Check sheet for the drawn part. Datum: minimum x, y, z corner. Units: mm. A direction names the side the tool comes from. Give positions to 0.01 mm unless a question says otherwise; leave off trailing zeros. Order: outer loops, then holes, each group sorted by start corner. A loop starts at its lowest first (then second) coordinate and runs counter-clockwise, first axis right, second up. Notation, with made-up numbers: (63.25, 52) -> (97.25, 52) arc R14 ccw to (97.25, 70) -> close; hole circle Ø8 at (2.5, 42). An arc over 180 degrees is marked (long way). One line per question, with ' | ' between items. Start each with the question number.
Q1. Section check A-A on x = 15. Record the cut outline in (y, z), plus the area to 3 significant figures.
Q2. Mould release check, pull along Z, two halves, no side actions. Record for the marked faces 4, 5 and 6: released by +Z, released by -Z, zero draft, split by the parting line, or undercut.
Q3. Section check B-B on x = 41.25. Record the cut outline in (y, z), plus the area to 3 significant figures.
Q4. Access from +Z, -Z, +X, -X, +Y, -Y to the whole of each face (thin tool, end or side, straight path). Record for the marked faces 1, 2 and 3.
Q5. Go/stop test with flat-tipped pins: pin 1 (11 mm diameter, centred on x = 15.5, y = 15, fed in from +Z); pin 2 (5 mm diameter, centred on x = 15, y = 13, fed in from +Z); pin 3 (5 mm diameter, centred on y = 38.5, z = 12, fed in from -X); pin 4 (12 mm diameter, centred on x = 38, z = 12, fed in from +Y). Record where each tip stops, or that it passes through.
Q6. Section check D-D on z = 10.25. Record the cut outline in (x, y), plus the area to 3 significant figures.
Q7. Material ranges on probe 1 along Y at (x, z) = (15, 1.55); probe 2 along Y at (x, z) = (15, 4.5); probe 3 along Y at (x, z) = (50.5, 6), recorded low to high. Write a range as [from, to].
Q8. Section check C-C on y = 13. Record the cut outline in (x, z).
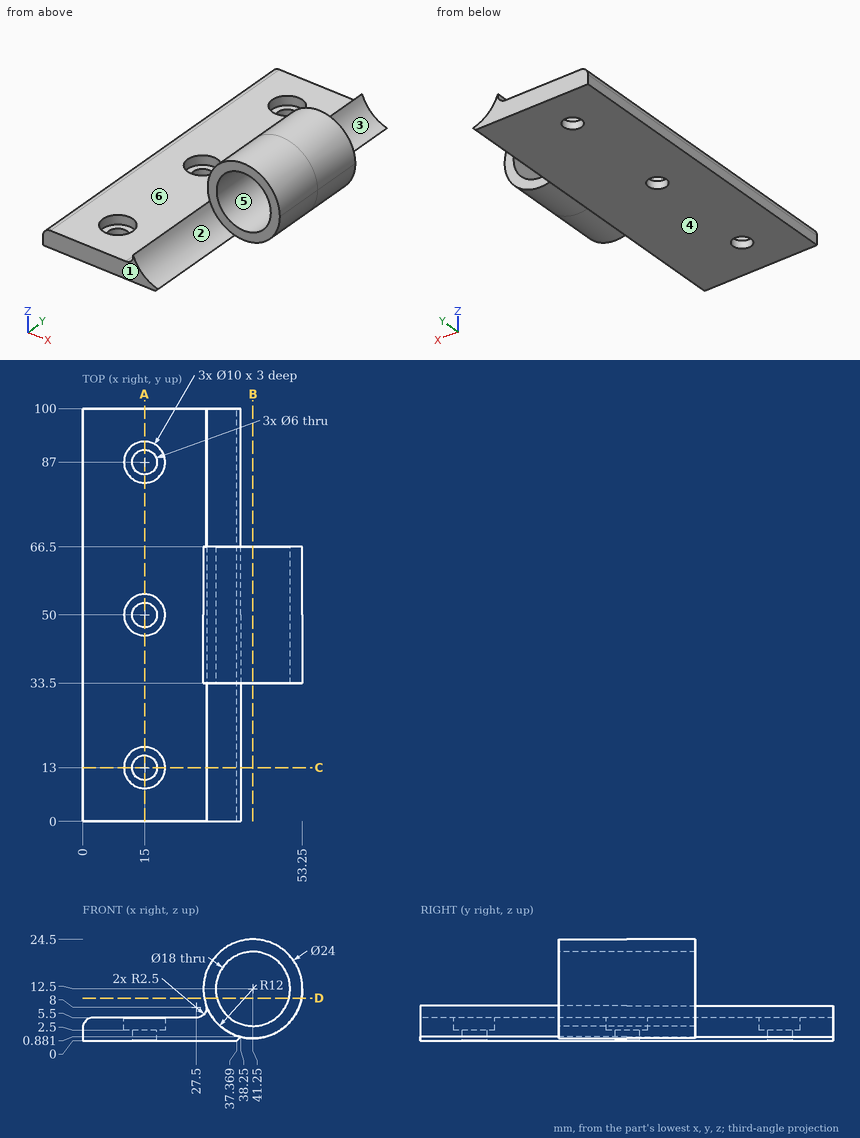
Filled in:
1) outline: (0, 0) -> (10, 0) -> (10, 2.5) -> (8, 2.5) -> (8, 5.5) -> (0, 5.5) -> close; (16, 0) -> (47, 0) -> (47, 2.5) -> (45, 2.5) -> (45, 5.5) -> (18, 5.5) -> (18, 2.5) -> (16, 2.5) -> close; (53, 0) -> (84, 0) -> (84, 2.5) -> (82, 2.5) -> (82, 5.5) -> (55, 5.5) -> (55, 2.5) -> (53, 2.5) -> close; (90, 0) -> (100, 0) -> (100, 5.5) -> (92, 5.5) -> (92, 2.5) -> (90, 2.5) -> close | area: 415 mm²
2) face 4: released by -Z | face 5: undercut | face 6: released by +Z
3) outline: (33.5, 0.5) -> (66.5, 0.5) -> (66.5, 3.5) -> (33.5, 3.5) -> close; (33.5, 21.5) -> (66.5, 21.5) -> (66.5, 24.5) -> (33.5, 24.5) -> close | area: 198 mm²
4) face 1: +Z, -Z, +X, -X, -Y | face 2: +Z, +X, -Y | face 3: +Z, +X, +Y
5) pin 1: z = 5.5 | pin 2: through | pin 3: x = 29.25 | pin 4: y = 66.5
6) outline: (29.46, 33.5) -> (32.54, 33.5) -> (32.54, 66.5) -> (29.46, 66.5) -> close; (49.96, 33.5) -> (53.04, 33.5) -> (53.04, 66.5) -> (49.96, 66.5) -> close | area: 203 mm²
7) probe 1: [0, 10], [16, 47], [53, 84], [90, 100] | probe 2: [0, 8], [18, 45], [55, 82], [92, 100] | probe 3: [33.5, 66.5]
8) outline: (0, 0) -> (12, 0) -> (12, 2.5) -> (10, 2.5) -> (10, 5.5) -> (2.5, 5.5) arc R2.5 ccw to (0, 3) -> close; (18, 0) -> (37.37, 0) -> (38.25, 0.88) arc R12 cw to (29.96, 8.42) arc R2.5 cw to (27.5, 5.5) -> (20, 5.5) -> (20, 2.5) -> (18, 2.5) -> close
